```python
from build123d import *

# Parameters (mm, degrees)
PAD_DEPTH    = 12.7
PAD001_DEPTH = 2.54


with BuildPart() as part:
    # Sketch → Pad (new body)
    with BuildSketch(Plane.XY):
        with BuildLine():
            Line((-25.273, -12.573), (-25.273, 12.573))
            ThreePointArc((-12.573, 25.273), (-21.553256, 21.553256), (-25.273, 12.573))
            Line((-12.573, 25.273), (12.573, 25.273))
            ThreePointArc((25.273, 12.573), (21.553256, 21.553256), (12.573, 25.273))
            Line((25.273, 12.573), (25.273, -12.573))
            ThreePointArc((12.573, -25.273), (21.553256, -21.553256), (25.273, -12.573))
            Line((12.573, -25.273), (-12.573, -25.273))
            ThreePointArc((-25.273, -12.573), (-21.553256, -21.553256), (-12.573, -25.273))
        make_face()
        with BuildLine():
            Line((-22.733, -12.573), (-22.733, 12.573))
            ThreePointArc((-12.573, 22.733), (-19.757205, 19.757205), (-22.733, 12.573))
            Line((-12.573, 22.733), (12.573, 22.733))
            ThreePointArc((22.733, 12.573), (19.757205, 19.757205), (12.573, 22.733))
            Line((22.733, 12.573), (22.733, -12.573))
            ThreePointArc((12.573, -22.733), (19.757205, -19.757205), (22.733, -12.573))
            Line((12.573, -22.733), (-12.573, -22.733))
            ThreePointArc((-22.733, -12.573), (-19.757205, -19.757205), (-12.573, -22.733))
        make_face(mode=Mode.SUBTRACT)
    extrude(amount=PAD_DEPTH)

    # Sketch001 → Pad001 (join)
    with BuildSketch(Plane.XY):
        with BuildLine():
            Line((-28.870723, -16.399415), (-28.870723, 16.399415))
            ThreePointArc((-16.399415, 28.870723), (-25.217961, 25.217961), (-28.870723, 16.399415))
            Line((-16.399415, 28.870723), (16.399415, 28.870723))
            ThreePointArc((28.870723, 16.399415), (25.217961, 25.217961), (16.399415, 28.870723))
            Line((28.870723, 16.399415), (28.870723, -16.399415))
            ThreePointArc((16.399415, -28.870723), (25.217961, -25.217961), (28.870723, -16.399415))
            Line((16.399415, -28.870723), (-16.399415, -28.870723))
            ThreePointArc((-28.870723, -16.399415), (-25.217961, -25.217961), (-16.399415, -28.870723))
        make_face()
    extrude(amount=-PAD001_DEPTH)


solid = part.part
```
Verification items for the finished model (mm, model axes). A direction names the side the tool comes from. Give positions to 0.01 mm unless a question says otherwise; leave off trailing zeros. Order: outer loops, then holes, each group sorted by start corner. A loop starts at its lowest first (then second) coordinate and runs counter-clockwise, first axis right, second up. Notation, with made-up numbers: M 38.5,71 L 76.5,71 A19 ccw 76.5,95 Z; hole C 10,28.25 d7. An arc over 180 degrees is marked long. Answer in a Markdown table with one row per item. Add a question column.
Item 1: Gauge pin test, flat ends, axial feed: pin 1 (1.5 mm diameter, centred on y = 9, z = 4.5, fed in from -X); pin 2 (12 mm diameter, centred on x = 10.5, y = -4, fed in from +Z); pin 3 (2 mm diameter, centred on x = 22, z = 6.5, fed in from -Y). Record the tip position at first contact, or that the pin passes through.
Item 2: Section check B-B, the plane x = -10.5. Enter the section's corners in (y, z), and give its area (3 significant figures).
Item 3: Mould release check, pull along X, two halves, no side actions. Record for faces 1 (the cylindrical face through (25.12, -25.314, -1.252)), 2 (the cylindrical face through (-19.836, -19.678, 6.261)), 3 (the flat face through (-25.273, 0, 6)), 4 (the flat face through (0, -28.871, -1)): released by +X, released by -X, zero draft, split by the parting line, or undercut.
Item 4: Tool access check on faces 5 (the flat face through (22.733, 0, 6)), 6 (the flat face through (0, -25.273, 6)), 7 (the cylindrical face through (21.651, 21.454, 6.261)), 8 (the cylindrical face through (-21.454, 21.651, 6.261)). Record the directions out of +Z, -Z, +X, -X, +Y, -Y that give a thin tool (end or side, any length) a straight path to the whole face; none if there is none.
Item 5: Scan lines: probe 1 along X at (y, z) = (-7.5, 8); probe 2 along Z at (x, y) = (2, -11). Record each from-to range of solid material in increasing order. Write a range as from..to.
Item 6: Section check D-D, the plane x = 24.5. Enter the section's corners in (y, z).
Item 7: Section check A-A, the plane z = 8.75. Enter the section's corners in (x, y), and give its area (3 significant figures).
Filled sheet:
| question | item | result |
|---|---|---|
| 1 | pin 1 | stops at x = -25.27 |
| 1 | pin 2 | stops at z = 0 |
| 1 | pin 3 | stops at y = -22.07 |
| 2 | outline | M -28.87,-2.54 L 28.87,-2.54 L 28.87,0 L 25.27,0 L 25.27,12.7 L 22.73,12.7 L 22.73,0 L -22.73,0 L -22.73,12.7 L -25.27,12.7 L -25.27,0 L -28.87,0 Z |
| 2 | area | 211 mm^2 |
| 3 | face 1 | released by +X |
| 3 | face 2 | undercut |
| 3 | face 3 | released by -X |
| 3 | face 4 | zero draft |
| 4 | face 5 | +Z |
| 4 | face 6 | +Z, +X, -X, -Y |
| 4 | face 7 | +Z, +X, +Y |
| 4 | face 8 | +Z, -X, +Y |
| 5 | probe 1 | x = -25.27..-22.73, 22.73..25.27 |
| 5 | probe 2 | z = -2.54..0 |
| 6 | outline | M -25.88,-2.54 L 25.88,-2.54 L 25.88,0 L 16.94,0 L 16.94,12.7 L -16.94,12.7 L -16.94,0 L -25.88,0 Z |
| 7 | outline | M -25.27,-12.57 A12.7 ccw -12.57,-25.27 L 12.57,-25.27 A12.7 ccw 25.27,-12.57 L 25.27,12.57 A12.7 ccw 12.57,25.27 L -12.57,25.27 A12.7 ccw -25.27,12.57 Z; hole M -22.73,-12.57 A10.16 ccw -12.57,-22.73 L 12.57,-22.73 A10.16 ccw 22.73,-12.57 L 22.73,12.57 A10.16 ccw 12.57,22.73 L -12.57,22.73 A10.16 ccw -22.73,12.57 Z |
| 7 | area | 438 mm^2 |
